Drawing for the job (mm, zero at the part's lowest x, y, z). A direction names the side the tool comes from. Give positions to 0.01 mm unless a question says otherwise; leave off trailing zeros. Write each loop counter-clockwise with the first axis right and the second up, starting at its lowest first coordinate (ties: lowest second). Pieces come first, ordered by that corner, then holes. Notation, with made-up numbers: M 0,55.5 L 43,55.5 A26 cw 43,79.5 Z; hole C -18,18.25 d9. An arc over 180 degrees is marked long. Answer as a JSON object with one key per item and string values. Group by question number.
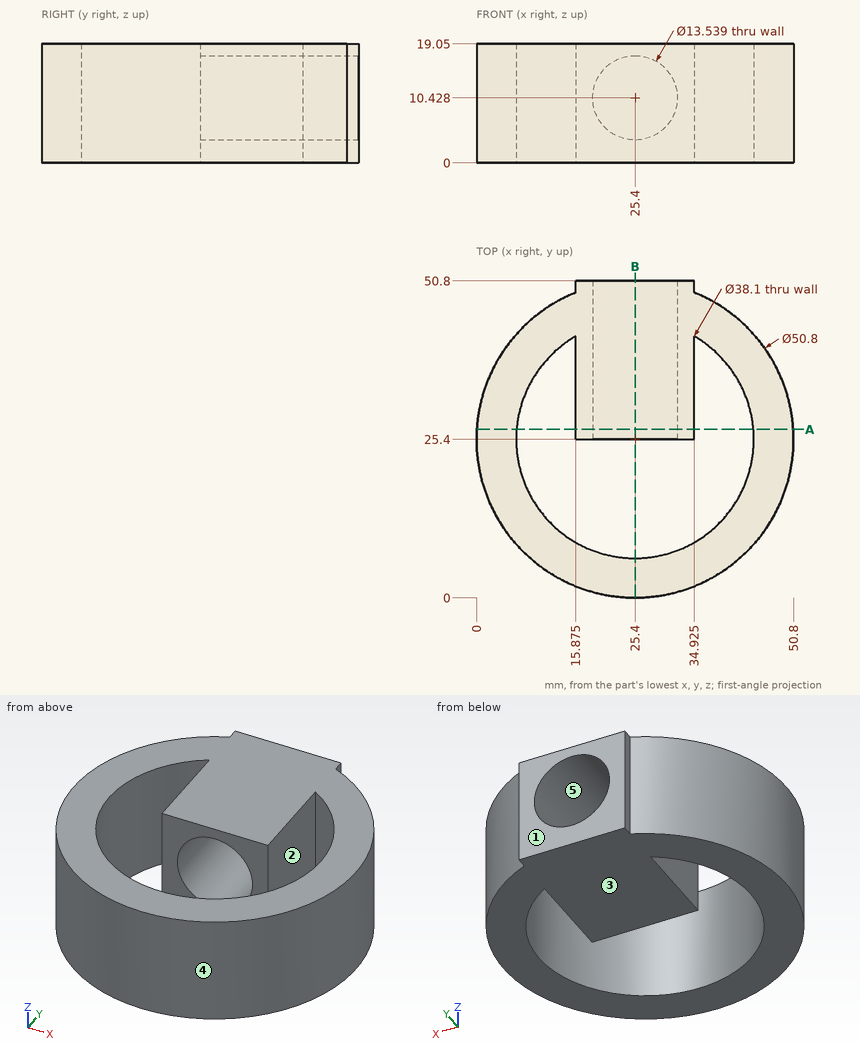
Q1. Slice it at A-A, the plane y = 27. Count the separate pieces of the cut face and the enclosed holes in it.
Q2. 3-axis set-ups, long thin cutter, end or side, ignore diameter. For the marked faces 1 and 2: which of +Z, -Z, +X, -X, +Y, -Y reach the whole face in a straight line?
Q3. Slice it at B-B, the plane x = 25.4. Write the cut outline in (y, z).
Q4. Two-plate mould, pull along X, no slides. Class the marked faces 3, 4 and 5: +X half, -X half, draft (parallel to the pull), parting line (faces both ways), or undercut.
Q5. Wall check: L1, parallel to X at y = 29.5, z = 8.25 (1 decimal); L2, parallel to X at y = 37.5, z = 7.75 (1 decimal); L3, parallel to Y at x = 38, z = 4.5 (1 decimal). Give the ranges that are in metal, low to high.
Q6. Drop flat-ended pins along their axis: P1, Ø4, axis at x = 25, z = 17, coming from the +Y side; P2, Ø4, axis at y = 39, z = 11, coming from the -X side; P3, Ø8, axis at y = 32, z = 13.5, coming from the +X side; P4, Ø6, axis at y = 23.5, z = 8, coming from the -X side. Give the stop position or say it passes through.
Solved:
{
 "1": {"separate pieces": "3", "enclosed holes": "1"},
 "2": {"face 1": "+Z, -Z, +X, -X, +Y", "face 2": "+Z, -Z"},
 "3": {"outline": "M 0,0 L 6.35,0 L 6.35,19.05 L 0,19.05 Z; M 25.4,0 L 50.8,0 L 50.8,3.66 L 25.4,3.66 Z; M 25.4,17.2 L 50.8,17.2 L 50.8,19.05 L 25.4,19.05 Z"},
 "4": {"face 3": "draft", "face 4": "parting line", "face 5": "undercut"},
 "5": {"L1": "x = 0.3 to 6.8, 15.9 to 19, 31.8 to 34.9, 44 to 50.5", "L2": "x = 3.1 to 10.7, 15.9 to 19.2, 31.6 to 34.9, 40.1 to 47.7", "L3": "y = 3.3 to 11.1, 39.7 to 47.5"},
 "6": {"P1": "stops at y = 50.8", "P2": "stops at x = 2.8", "P3": "stops at x = 50.67", "P4": "stops at x = 0"}
}
